Can you work these out from the model? Positions are in its coordinate system, mm. Face numbers are marked on the shaded views. Give positions to 0.01 mm unless a question says otherwise; leave off trailing zeros. Loops run counter-clockwise (first coordinate to the right, second up) from the corner with the lowest first, then second, coordinate; pieces in that order, holes last. Notation, with made-up numbers: M 14.5,63 L 65.5,63 A18 cw 65.5,89 Z; hole C -16,-19 d11. An arc over 180 degrees is marked long. Put each result on its own line as item: value. Start each with the question number.
1) Imagine slicing it at A-A (y = 0). Write out the boundary of the cut face in (x, z) (3 decimals).
2) Imagine slicing it at D-D (y = 8.75). Write out the boundary of the cut face in (x, z).
3) Imagine slicing it at C-C (z = 36.5). Write out the boundary of the cut face in (x, y) (3 decimals).
4) Please list where these lines run through material, in increasing order: line 1 along X through (y, z) = (0, 32) (3 decimals); line 2 along Y through (x, z) = (-4, 19) (3 decimals); line 3 along Z through (x, y) = (-13, 2.75). Write a range as from..to.
5) For P1, Ø8, axis at x = -10.5, z = 29.5, coming from the -Y side (3 decimals), with a flat end and sliding along its axis, tell me the tip position at first contact or that it passes through.
6) Imagine slicing it at B-B (x = 0). Write out the boundary of the cut face in (y, z) (3 decimals), then the cut area to 3 significant figures.
7) If we mould it in two halves opening along Y, with no side actions, what happens to the marked faces 1, 2 and 3? For each: +Y half, -Y half, draft (parallel to the pull), parting line (faces both ways), or undercut.
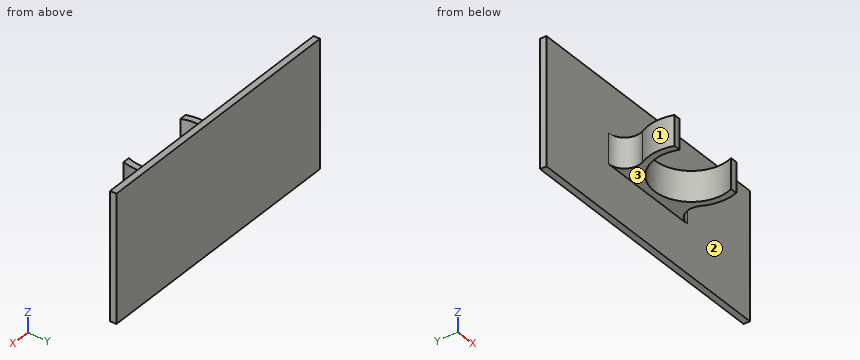
from build123d import *

# Parameters (mm, degrees)
SKETCH1_R           = 11.125
SKETCH1_R_2         = 9.125
BOSS_EXTRUDE1_DEPTH = 10
BOSS_EXTRUDE2_START = -10
BOSS_EXTRUDE2_DEPTH = 10
BOSS_EXTRUDE3_DEPTH = 40
SKETCH4_W           = 57.687127484
SKETCH4_H           = 15.25
SKETCH4_W_2         = 54.293767044
CUT_EXTRUDE1_DEPTH  = 42
SKETCH5_W           = 53.119142276
SKETCH5_H           = 26.885855795
CUT_EXTRUDE2_DEPTH  = 61


with BuildPart() as part:
    # Sketch1 → Boss-Extrude1 (new body)
    with BuildSketch(Plane.XY):
        Circle(SKETCH1_R)
        Circle(SKETCH1_R_2, mode=Mode.SUBTRACT)
    extrude(amount=BOSS_EXTRUDE1_DEPTH)

    # Sketch2 → Boss-Extrude2 (add)
    with BuildSketch(Plane.XY.offset(10).offset(BOSS_EXTRUDE2_START)):
        with BuildLine():
            Line((-9.125, -9.125), (-6.363961031, -9.125))
            ThreePointArc((-6.363961031, -9.125), (-7.866562941, -7.866562941), (-9.125, -6.363961031))
            Line((-9.125, -6.363961031), (-9.125, -9.125))
        make_face()
        with BuildLine():
            Line((-9.125, -11.125), (0, -11.125))
            ThreePointArc((0, -11.125), (-3.335416016, -10.613228774), (-6.363961031, -9.125))
            Line((-6.363961031, -9.125), (-9.125, -9.125))
            Line((-9.125, -9.125), (-9.125, -11.125))
        make_face()
        with BuildLine():
            Line((0, -11.125), (9.125, -11.125))
            Line((9.125, -11.125), (9.125, -9.125))
            Line((9.125, -9.125), (6.363961031, -9.125))
            ThreePointArc((6.363961031, -9.125), (3.335416016, -10.613228774), (0, -11.125))
        make_face()
        with BuildLine():
            Line((6.363961031, -9.125), (9.125, -9.125))
            Line((9.125, -9.125), (9.125, -6.363961031))
            ThreePointArc((9.125, -6.363961031), (7.866562941, -7.866562941), (6.363961031, -9.125))
        make_face()
    extrude(amount=BOSS_EXTRUDE2_DEPTH)

    # Sketch5 → Cut-Extrude2 (cut)
    with BuildSketch(Plane.XZ.offset(-13.625)):
        with Locations((1.239881699, 2.094817028)):
            Rectangle(SKETCH5_W, SKETCH5_H)
    extrude(amount=CUT_EXTRUDE2_DEPTH, mode=Mode.SUBTRACT)


with BuildPart() as body_2:
    # Sketch3 → Boss-Extrude3 (new body)
    with BuildSketch(Plane.XY.offset(10)):
        with BuildLine():
            Line((12.903487901, -4.375), (10.770329614, -4.375))
            ThreePointArc((10.770329614, -4.375), (0, 11.625), (-10.770329614, -4.375))
            Line((-10.770329614, -4.375), (-12.903487901, -4.375))
            ThreePointArc((-12.903487901, -4.375), (-13.584322253, 1.05205225), (-12.076010524, 6.309563758))
            ThreePointArc((-12.076010524, 6.309563758), (-12.231057843, 11.215638801), (-16.507574019, 13.625))
            Line((-16.507574019, 13.625), (-42.5, 13.625))
            Line((-42.5, 13.625), (-42.5, 15.625))
            Line((-42.5, 15.625), (42.5, 15.625))
            Line((42.5, 15.625), (42.5, 13.625))
            Line((42.5, 13.625), (16.507574019, 13.625))
            ThreePointArc((16.507574019, 13.625), (12.231057843, 11.215638801), (12.076010524, 6.309563758))
            ThreePointArc((12.076010524, 6.309563758), (13.584322253, 1.05205225), (12.903487901, -4.375))
        make_face()
    extrude(amount=BOSS_EXTRUDE3_DEPTH)

    # Sketch4 → Cut-Extrude1 (cut)
    with BuildSketch(Plane.XZ.offset(-13.625)):
        with Locations((1.827194083, 42.375)):
            Rectangle(SKETCH4_W, SKETCH4_H)
        with Locations((0.130513863, 17.625)):
            Rectangle(SKETCH4_W_2, SKETCH4_H)
    extrude(amount=CUT_EXTRUDE1_DEPTH, mode=Mode.SUBTRACT)


solid = body_2.part
Recorded:
1. outline: M -13.625,25.25 L -11.625,25.25 L -11.625,34.75 L -13.625,34.75 Z; M 11.625,25.25 L 13.625,25.25 L 13.625,34.75 L 11.625,34.75 Z
2. outline: M -11.51,25.25 L -7.65,25.25 L -7.65,34.75 L -11.51,34.75 Z; M 7.65,25.25 L 11.51,25.25 L 11.51,34.75 L 7.65,34.75 Z
3. outline: M -42.5,13.625 L 42.5,13.625 L 42.5,15.625 L -42.5,15.625 Z
4. line 1: -13.625..-11.625, 11.625..13.625
4. line 2: 13.625..15.625
4. line 3: 25.25..34.75
5. P1: y = -4.375
6. outline: M 11.625,25.25 L 13.625,25.25 L 13.625,10 L 15.625,10 L 15.625,50 L 13.625,50 L 13.625,34.75 L 11.625,34.75 Z
6. area: 99.0 mm²
7. face 1: undercut
7. face 2: -Y half
7. face 3: draft
